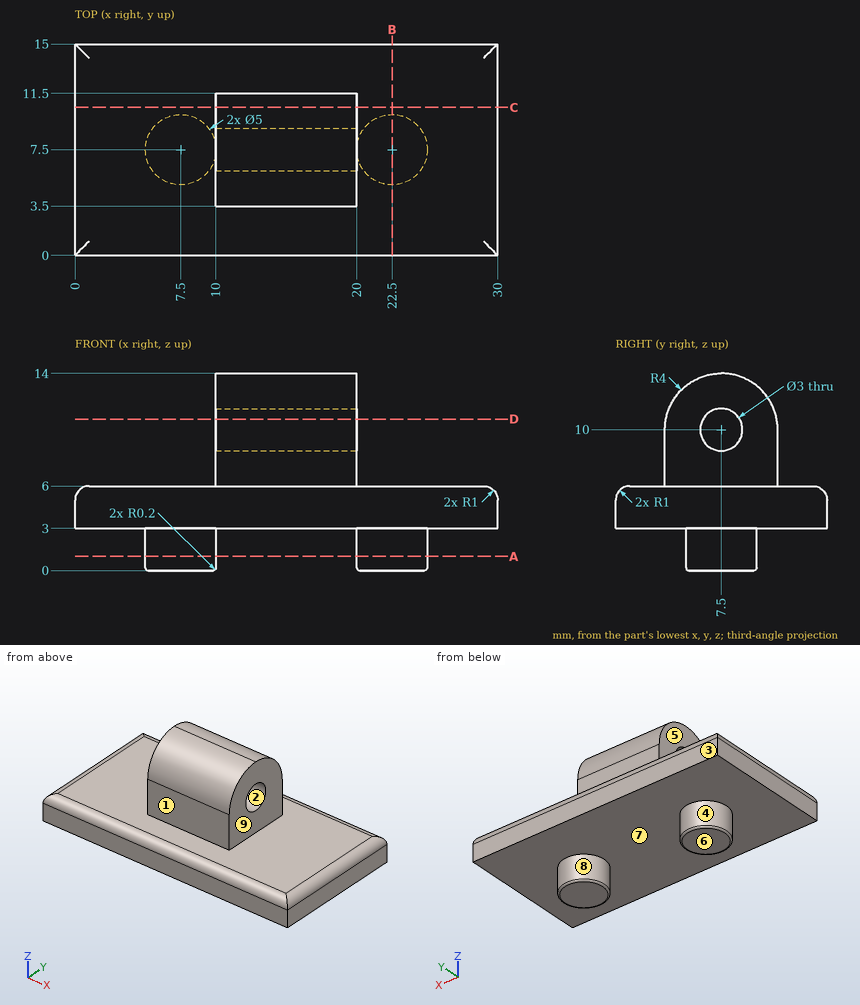
The figure shows three views and two pictorial views of one solid part (mm, origin at its lowest corner). Answer the questions. A direction names the side the tool comes from. Round coordinates to 2 decimals unless told otherwise and drop trailing zeros. Loops run counter-clockwise (first coordinate to the right, second up) from the corner with the lowest first, then second, coordinate; pieces in that order, holes last. Notation, with made-up numbers: (78, -6) -> (112, -6) arc R16 ccw to (112, 6) -> close; hole circle Ø1 at (-28, 49). An arc over 180 degrees is marked (long way). Use one line per item in the form item = value.
(1) Find section A-A on z = 1. Give the vertices of the cut face in (x, y), then the cut area to 3 significant figures.
Answer list:
outline = circle Ø5 at (7.5, 7.5); circle Ø5 at (22.5, 7.5)
area = 39.3 mm2
(2) Straight lines are drawn through the part: line 1 (Z direction, x = 16, y = 7.5); line 2 (X direction, y = 5.75, z = 11.75); line 3 (Z direction, x = 16.75, y = 1). For each, find the intervals that lie inside material, in ascending order.
Answer list:
line_1 = 3 to 8.5, 11.5 to 14
line_2 = 10 to 20
line_3 = 3 to 6
(3) Find section D-D on z = 10.75. Give the vertices of the cut face in (x, y).
Answer list:
outline = (10, 3.57) -> (20, 3.57) -> (20, 6.2) -> (10, 6.2) -> close; (10, 8.8) -> (20, 8.8) -> (20, 11.43) -> (10, 11.43) -> close
(4) For a pull along X with two mould halves and no side action, classify the marked faces 6, 7, 8 and 9 as released by +X, released by -X, zero draft, split by the parting line, or undercut.
Answer list:
face_6 = zero draft
face_7 = undercut
face_8 = undercut
face_9 = released by +X
(5) A tool of negligible diameter and unlimited length cuts with its end or side. For the marked faces 1, 2, 3, 4 and 5, from which of +Z, -Z, +X, -X, +Y, -Y can it reach the whole face along a straight path? Write none if from no direction.
Answer list:
face_1 = +Z, +X, -X, -Y
face_2 = +X, -X
face_3 = +Z, -Z, +X, -X, +Y
face_4 = -Z
face_5 = +Z, -X, +Y, -Y
(6) Flat-ended cylindrical pins translate along their axes: P1, Ø5, axis at x = 20, y = 13, coming from the +Z side; P2, Ø1.2, axis at x = 14.5, z = 8, coming from the +Y side; P3, Ø3, axis at x = 25, y = 8.5, coming from the +Z side; P4, Ø1.8, axis at y = 7.5, z = 10, coming from the -X side. Find the tip coordinate at first contact, or state that the pin passes through.
Answer list:
P1 = 12.65
P2 = 11.5
P3 = 6
P4 = through
(7) Find section C-C on y = 10.5. Give the vertices of the cut face in (x, z).
Answer list:
outline = (0, 3) -> (30, 3) -> (30, 5) arc R1 ccw to (29, 6) -> (20, 6) -> (20, 12.65) -> (10, 12.65) -> (10, 6) -> (1, 6) arc R1 ccw to (0, 5) -> close
(8) Find section B-B on x = 22.5. Give the vertices of the cut face in (y, z).
Answer list:
outline = (0, 3) -> (5, 3) -> (5, 0.2) arc R0.2 ccw to (5.2, 0) -> (9.8, 0) arc R0.2 ccw to (10, 0.2) -> (10, 3) -> (15, 3) -> (15, 5) arc R1 ccw to (14, 6) -> (1, 6) arc R1 ccw to (0, 5) -> close
